from build123d import *

# Parameters (mm, degrees)
SKETCH_R        = 5.5
SKETCH_R_2      = 4.1
SKETCH_W        = 11
SKETCH_H        = 10.5
PAD_DEPTH       = 2
SKETCH001_W     = 16.5
SKETCH001_H     = 16.5
PAD001_DEPTH    = 12.5
SKETCH002_W     = 140.5
SKETCH002_H     = 3
PAD002_DEPTH    = 17
SKETCH003_W     = 16.5
SKETCH003_H     = 10
PAD003_DEPTH    = 15
SKETCH004_R     = 1.65
POCKET_DEPTH    = 20
POCKET001_DEPTH = 3.5
SKETCH006_R     = 1.6
POCKET002_DEPTH = 20
POCKET003_DEPTH = 3
SKETCH008_R     = 1.6
POCKET004_DEPTH = 5
POCKET005_DEPTH = 2.8
POCKET006_DEPTH = 2.8
CHAMFER_SIZE    = 0.8
CHAMFER001_SIZE = 1
SKETCH011_W     = 142.26446
SKETCH011_H     = 19.063439
POCKET007_DEPTH = 1
FILLET_R        = 2
FILLET001_R     = 2
FILLET002_R     = 2
FILLET003_R     = 2
FILLET004_R     = 2
FILLET005_R     = 1
FILLET006_R     = 1
FILLET007_R     = 0.5


with BuildPart() as part:
    # Sketch → Pad (new body)
    with BuildSketch(Plane.XY):
        Polygon((0, 19), (131, 19), (131, 0), (0, 0), (-9.5, 0), (-9.5, 19), align=None)
        with Locations((15.25, 9.25)):
            Circle(SKETCH_R, mode=Mode.SUBTRACT)
        with Locations((29.75, 9.25)):
            Circle(SKETCH_R, mode=Mode.SUBTRACT)
        with Locations((44.25, 9.25)):
            Circle(SKETCH_R, mode=Mode.SUBTRACT)
        with Locations((58.75, 9.25)):
            Circle(SKETCH_R, mode=Mode.SUBTRACT)
        with Locations((108, 9.25)):
            Circle(SKETCH_R_2, mode=Mode.SUBTRACT)
        with Locations((123, 9.25)):
            Circle(SKETCH_R_2, mode=Mode.SUBTRACT)
        with Locations((95, 7.75)):
            Rectangle(SKETCH_W, SKETCH_H, mode=Mode.SUBTRACT)
    extrude(amount=PAD_DEPTH)

    # Sketch001 → Pad001 (new body)
    with BuildSketch(Plane.XY.offset(2)):
        with Locations((-1.25, 10.75)):
            Rectangle(SKETCH001_W, SKETCH001_H)
        Polygon((63.25, 19), (72.75, 19), (72.75, 2.5), (65.5, 2.5), (65.5, 16), (63.25, 16), align=None)
    extrude(amount=-PAD001_DEPTH)

    # Sketch002 → Pad002 (new body)
    with BuildSketch(Plane.XY.offset(2)):
        with Locations((60.75, 17.5)):
            Rectangle(SKETCH002_W, SKETCH002_H)
    extrude(amount=-PAD002_DEPTH)

    # Sketch003 → Pad003 (new body)
    with BuildSketch(Plane(origin=(0, 0, 0), x_dir=(1, 0, 0), z_dir=(0, 0, -1))):
        with Locations((-1.25, -14)):
            Rectangle(SKETCH003_W, SKETCH003_H)
    extrude(amount=PAD003_DEPTH)

    # Sketch004 → Pocket (cut)
    with BuildSketch(Plane.XZ.offset(-2.5)):
        with Locations((3, -6)):
            Circle(SKETCH004_R)
        with Locations((68, -6)):
            Circle(SKETCH004_R)
    extrude(amount=-POCKET_DEPTH, mode=Mode.SUBTRACT)

    # Sketch005 → Pocket001 (cut)
    with BuildSketch(Plane(origin=(0, 19, 0), x_dir=(-1, 0, 0), z_dir=(0, 1, 0))):
        Polygon((-4.802997, -3.386088), (-6.165213, -6.254486), (-4.362215, -8.868397), (-1.197003, -8.613912), (0.165213, -5.745514), (-1.637785, -3.131603), align=None)
        Polygon((-64.831829, -5.78546), (-66.601711, -3.149014), (-69.769882, -3.363554), (-71.168171, -6.21454), (-69.398289, -8.850986), (-66.230118, -8.636446), align=None)
    extrude(amount=-POCKET001_DEPTH, mode=Mode.SUBTRACT)

    # Sketch006 → Pocket002 (cut)
    with BuildSketch(Plane(origin=(-9.5, 0, 0), x_dir=(0, -1, 0), z_dir=(-1, 0, 0))):
        with Locations((-12.58756, -10)):
            Circle(SKETCH006_R)
    extrude(amount=-POCKET002_DEPTH, mode=Mode.SUBTRACT)

    # Sketch007 → Pocket003 (cut)
    with BuildSketch(Plane.YZ.offset(7)):
        Polygon((14.285865, -12.886017), (15.936076, -9.972234), (14.237772, -7.086217), (10.889255, -7.113983), (9.239044, -10.027766), (10.937348, -12.913783), align=None)
    extrude(amount=-POCKET003_DEPTH, mode=Mode.SUBTRACT)

    # Sketch008 → Pocket004 (cut)
    with BuildSketch(Plane.XY.offset(2)):
        with Locations((69.12, 5.7)):
            Circle(SKETCH008_R)
        with Locations((-1.01165, 5.7)):
            Circle(SKETCH008_R)
    extrude(amount=-POCKET004_DEPTH, mode=Mode.SUBTRACT)

    # Sketch009 → Pocket005 (cut)
    with BuildSketch(Plane(origin=(0, 0, 0), x_dir=(1, 0, 0), z_dir=(0, 0, -1))):
        Polygon((66.259544, -7.723634), (69.163413, -9.350056), (72.023869, -7.648441), (72.023869, -2.059704), (66.259544, -2.059704), align=None)
    extrude(amount=POCKET005_DEPTH, mode=Mode.SUBTRACT)

    # Sketch010 → Pocket006 (cut)
    with BuildSketch(Plane(origin=(0, 0, 0), x_dir=(1, 0, 0), z_dir=(0, 0, -1))):
        Polygon((-3.837748, -7.811181), (-0.999162, -9.409884), (1.845776, -7.757931), (1.845776, -1.91964), (-3.837748, -1.91964), align=None)
    extrude(amount=POCKET006_DEPTH, mode=Mode.SUBTRACT)

    # Chamfer
    chamfer_edges = [part.edges().sort_by_distance(p)[0] for p in [
        (66.35, 15.5, -6),
    ]]
    chamfer(chamfer_edges, length=CHAMFER_SIZE)

    # Chamfer001
    chamfer001_edges = [part.edges().sort_by_distance(p)[0] for p in [
        (1.35, 15.5, -6),
    ]]
    chamfer(chamfer001_edges, length=CHAMFER001_SIZE)

    # Sketch011 → Pocket007 (cut)
    with BuildSketch(Plane(origin=(0, 19, 0), x_dir=(-1, 0, 0), z_dir=(0, 1, 0))):
        with Locations((-60.301471, -6.813256)):
            Rectangle(SKETCH011_W, SKETCH011_H)
    extrude(amount=-POCKET007_DEPTH, mode=Mode.SUBTRACT)

    # Fillet
    fillet_edges = [part.edges().sort_by_distance(p)[0] for p in [
        (72.75, 9.25, -10.5),
    ]]
    fillet(fillet_edges, radius=FILLET_R)

    # Fillet001
    fillet001_edges = [part.edges().sort_by_distance(p)[0] for p in [
        (65.5, 9.25, -10.5),
    ]]
    fillet(fillet001_edges, radius=FILLET001_R)

    # Fillet002
    fillet002_edges = [part.edges().sort_by_distance(p)[0] for p in [
        (131, 0, 1),
    ]]
    fillet(fillet002_edges, radius=FILLET002_R)

    # Fillet003
    fillet003_edges = [part.edges().sort_by_distance(p)[0] for p in [
        (131, 17, -15),
    ]]
    fillet(fillet003_edges, radius=FILLET003_R)

    # Fillet004
    fillet004_edges = [part.edges().sort_by_distance(p)[0] for p in [
        (-9.5, 0, 1),
    ]]
    fillet(fillet004_edges, radius=FILLET004_R)

    # Fillet005
    fillet005_edges = [part.edges().sort_by_distance(p)[0] for p in [
        (101.875, 16, 0),
    ]]
    fillet(fillet005_edges, radius=FILLET005_R)

    # Fillet006
    fillet006_edges = [part.edges().sort_by_distance(p)[0] for p in [
        (35.125, 16, 0),
    ]]
    fillet(fillet006_edges, radius=FILLET006_R)

    # Fillet007
    fillet007_edges = [part.edges().sort_by_distance(p)[0] for p in [
        (65.5, 8.75, 0),
    ]]
    fillet(fillet007_edges, radius=FILLET007_R)


solid = part.part
For this review, take the finished solid that the model builds, in its own axes (mm). A direction names the side the tool comes from. Give positions to 0.01 mm unless a question says otherwise; leave off trailing zeros. Loops run counter-clockwise (first coordinate to the right, second up) from the corner with the lowest first, then second, coordinate; pieces in that order, holes last.
Item 1: For line 1 along Z through (x, y) = (67, 5.75); line 2 along Z through (x, y) = (68, 8.75); line 3 along Y through (x, z) = (15.25, 0.9), list the stretches that pass through material, from the lowest coordinate up.
Item 2: Tool access review of faces 4 (the flat face through (70.574, 8.511, -1.38)), 5 (the flat face through (5.52, 15.1, -11.45)), 6 (the flat face through (0.525, 16.768, -7.2)): name each direction out of +Z, -Z, +X, -X, +Y, -Y from which nothing blocks a thin tool from reaching the whole face with its end or side.
Item 3: Insertion check: pin 1 (5 mm diameter, centred on y = 9.5, z = -7.5, fed in from +X); pin 2 (2 mm diameter, centred on x = 88, y = 7, fed in from -Z); pin 3 (2.5 mm diameter, centred on x = 69.12, y = 5.7, fed in from +Z). Each pin has a flat end and moves straight along its axis. Give the tip position at first contact, or say it passes through.
Item 4: Draft analysis for pull direction Z (two halves, no side actions). For faces 1 (the cylindrical face through (-1.22, 7.286, 1.014)), 2 (the flat face through (-1, 6, -10.5)), 3 (the flat face through (-3.838, 5, -1)), state which applies: +Z half, -Z half, draft (parallel to the pull), parting line (faces both ways), or undercut.
Item 5: Take a section at B-B, the plane x = 81.5. State the section outline as (y, z) points, and give its area (3 significant figures).
Item 6: Take a section at A-A, the plane x = 15.25. State the section outline as (y, z) points, and give its area (3 significant figures).
Item 7: Take a section at C-C, the plane x = 123. State the section outline as (y, z) points.
Calculated:
1. line 1: z = -10.44 to -7.31, -4.69 to -2.8, 0 to 2
1. line 2: z = -10.5 to -7.65, -4.35 to 2
1. line 3: y = 0 to 3.75, 14.75 to 18
2. face 4: -Y
2. face 5: none
2. face 6: +Y
3. pin 1: stops at x = 72.75
3. pin 2: stops at z = 0
3. pin 3: stops at z = -3
4. face 1: draft
4. face 2: -Z half
4. face 3: undercut
5. outline: (0, 0) - (15, 0) arc R1 cw to (16, -1) - (16, -15) - (18, -15) - (18, 2) - (0, 2) - close
5. area: 66.2 mm2
6. outline: (0, 0) - (3.75, 0) - (3.75, 2) - (0, 2) - close; (14.75, 0) - (15, 0) arc R1 cw to (16, -1) - (16, -15) - (18, -15) - (18, 2) - (14.75, 2) - close
6. area: 44.2 mm2
7. outline: (0, 0) - (5.15, 0) - (5.15, 2) - (0, 2) - close; (13.35, 0) - (15, 0) arc R1 cw to (16, -1) - (16, -15) - (18, -15) - (18, 2) - (13.35, 2) - close
